Here's how the part is built. I have some questions about the finished solid (model axes, mm). A direction names the side the tool comes from. Coordinates: 2 decimals unless noted, no trailing zeros. Write each loop counter-clockwise with the first axis right and the second up, starting at its lowest first coordinate (ties: lowest second). Pieces come first, ordered by that corner, then holes. Notation, with made-up numbers: M 65,69 L 114,69 A23 cw 114,105 Z; hole C -10,75.5 d11. An arc over 180 degrees is marked long. Use one line per item in the form item = value. Start each with the question number.
1. I'm going to push flat-ended pins straight in: pin 1 Ø2 at (x, y) = (0, -12) entering from -Z; pin 2 Ø7 at (x, y) = (48.02, -4.9) entering from -Z; pin 3 Ø8 at (x, z) = (13.5, 28.5) entering from +Y. Where does each tip first touch, or does it pass through?
2. I want a section at D-D, the plane z = 19. List the corners of the cut face in (x, y) for me.
3. I want a section at C-C, the plane x = 3. List the corners of the cut face in (y, z) for me, plus the area to 3 significant figures.
4. Thinking about a two-plate mould opening in X: for faces 5 (the face through (-0.08, 6.57, 36.01)), 6 (the face through (0.91, -0.6, 31.42)), 7 (the face through (18.214, 6.843, 36.012)), which applies, released by +X, released by -X, zero draft, split by the parting line, or undercut?
5. On a 3-axis mill with a long thin cutter (end or side, diameter ignored), from which of +Z, -Z, +X, -X, +Y, -Y can I reach the whole of each face in a straight line? I mean faces 1 (the face through (47, -11, 31.991)), 2 (the face through (12, 2.5, 27)), 3 (the face through (4.118, 5, 31)), 4 (the face through (4.118, -10, 34)). Say none if no direction works.
6. Please list where these lines run through material, in increasing order: line 1 along X through (y, z) = (-4, 33); line 2 along Y through (x, z) = (29.5, 28.5); line 3 along Z through (x, y) = (44.5, -13.5). Write a range as [from, to].
7. I want a section at B-B, the plane y = -4.9. List the corners of the cut face in (x, z) for me, plus the area to 3 significant figures.
8. I want a section at A-A, the plane y = -12. List the corners of the cut face in (x, z) for me, plus the area to 3 significant figures.
from build123d import *

# Parameters (mm, degrees)
SKETCH1_W                = 53
SKETCH1_H                = 30.745586227
BOSS_EXTRUDE1_DEPTH      = 3
SKETCH2_W                = 6.5
SKETCH2_H                = 3
BOSS_EXTRUDE2_DEPTH      = 20
SKETCH3_R                = 2.15
CUT_EXTRUDE1_DEPTH       = 3
SKETCH6_W                = 17
SKETCH6_H                = 7.58
BOSS_EXTRUDE3_DEPTH      = 3
SKETCH7_R                = 1.5
CUT_EXTRUDE2_DEPTH       = 7.5
SKETCH8_W                = 6
SKETCH8_H                = 14
CUT_EXTRUDE3_DEPTH       = 0.5
FILLET1_R                = 2
BOSS_EXTRUDE4_DEPTH      = 2
BOSS_EXTRUDE4_DEPTH_BACK = 2
BOSS_EXTRUDE5_DEPTH      = 3


with BuildPart() as part:
    # Sketch1 → Boss-Extrude1 (new body)
    with BuildSketch(Plane(origin=(0, 0, 0), x_dir=(1, 0, 0), z_dir=(0, 1, 0))):
        with Locations((24.118089155, -22.118099476)):
            Rectangle(SKETCH1_W, SKETCH1_H)
    extrude(amount=BOSS_EXTRUDE1_DEPTH)

    # Sketch2 → Boss-Extrude2 (add)
    with BuildSketch(Plane.XZ):
        with Locations((47.368089155, 33.49089259)):
            Rectangle(SKETCH2_W, SKETCH2_H)
        with Locations((0.868089155, 33.49089259)):
            Rectangle(SKETCH2_W, SKETCH2_H)
    extrude(amount=BOSS_EXTRUDE2_DEPTH)

    # Sketch3 → Cut-Extrude1 (cut)
    with BuildSketch(Plane.XY.offset(34.99089259)):
        with Locations((48.018089155, -15.1)):
            Circle(SKETCH3_R)
        with Locations((48.018089155, -4.9)):
            Circle(SKETCH3_R)
        with Locations((0.218089155, -15.1)):
            Circle(SKETCH3_R)
        with Locations((0.218089155, -4.9)):
            Circle(SKETCH3_R)
    extrude(amount=-CUT_EXTRUDE1_DEPTH, mode=Mode.SUBTRACT)

    # Sketch6 → Boss-Extrude3 (add)
    with BuildSketch(Plane.XY.offset(37.49089259)):
        with Locations((6.118089155, 6.79)):
            Rectangle(SKETCH6_W, SKETCH6_H)
    extrude(amount=-BOSS_EXTRUDE3_DEPTH)

    # Sketch7 → Cut-Extrude2 (cut)
    with BuildSketch(Plane.XY.offset(37.49089259)):
        with Locations((0.118089155, 5.081241932)):
            Circle(SKETCH7_R)
        with Locations((11.618089155, 5.081241932)):
            Circle(SKETCH7_R)
    extrude(amount=-CUT_EXTRUDE2_DEPTH, mode=Mode.SUBTRACT)

    # Sketch8 → Cut-Extrude3 (cut)
    with BuildSketch(Plane(origin=(0, 3, 0), x_dir=(1, 0, 0), z_dir=(0, 1, 0))):
        with Locations((11.618089155, -27.49089259)):
            Rectangle(SKETCH8_W, SKETCH8_H)
        with Locations((0.618089155, -27.49089259)):
            Rectangle(SKETCH8_W, SKETCH8_H)
    extrude(amount=-CUT_EXTRUDE3_DEPTH, mode=Mode.SUBTRACT)

    # Fillet1
    fillet1_edges = [part.edges().sort_by_distance(p)[0] for p in [
        (47.368089155, 0, 31.99089259),
        (0.868089155, 0, 31.99089259),
    ]]
    fillet(fillet1_edges, radius=FILLET1_R)

    # Sketch13 → Boss-Extrude4 (add, two sides: drawn at the far end of the back side and taken through both)
    with BuildSketch(Plane.ZY.offset(-6.118089155).offset(-BOSS_EXTRUDE4_DEPTH_BACK)):
        Polygon((34.49089259, 10.57033397), (34.49089259, 3), (20.468920989, 3), align=None)
    extrude(amount=BOSS_EXTRUDE4_DEPTH + BOSS_EXTRUDE4_DEPTH_BACK)

    # Sketch14 → Boss-Extrude5 (add)
    with BuildSketch(Plane.XY.offset(37.49089259)):
        Polygon((14.618089155, 3), (14.618089155, 10.58), (21.91210821, 3), align=None)
    extrude(amount=-BOSS_EXTRUDE5_DEPTH)


solid = part.part
Answer list:
q1.pin_1 = 31.99
q1.pin_2 = 31.9
q1.pin_3 = 3
q2.outline = M -2.38,0 L 50.62,0 L 50.62,3 L -2.38,3 Z
q3.outline = M -20,31.99 L -2,31.99 A2 cw 0,29.99 L 0,6.75 L 3,6.75 L 3,20.49 L 2.5,20.49 L 2.5,34.49 L 10.58,34.49 L 10.58,37.49 L 0,37.49 L 0,34.99 L -20,34.99 Z
q3.area = 169 mm²
q4.face_5 = undercut
q4.face_6 = zero draft
q4.face_7 = released by +X
q5.face_1 = -Z, +X, -X, -Y
q5.face_2 = +Y
q5.face_3 = -Z, -X, +Y
q5.face_4 = +Z, -Z, -Y
q6.line_1 = [-2.38, -1.73], [2.17, 4.12], [44.12, 46.07], [49.97, 50.62]
q6.line_2 = [0, 3]
q6.line_3 = [31.99, 34.99]
q7.outline = M -2.38,31.99 L -1.93,31.99 L -1.93,34.99 L -2.38,34.99 Z; M 2.37,31.99 L 4.12,31.99 L 4.12,34.99 L 2.37,34.99 Z; M 44.12,31.99 L 45.87,31.99 L 45.87,34.99 L 44.12,34.99 Z; M 50.17,31.99 L 50.62,31.99 L 50.62,34.99 L 50.17,34.99 Z
q7.area = 13.2 mm²
q8.outline = M -2.38,31.99 L 4.12,31.99 L 4.12,34.99 L -2.38,34.99 Z; M 44.12,31.99 L 50.62,31.99 L 50.62,34.99 L 44.12,34.99 Z
q8.area = 39.0 mm²
